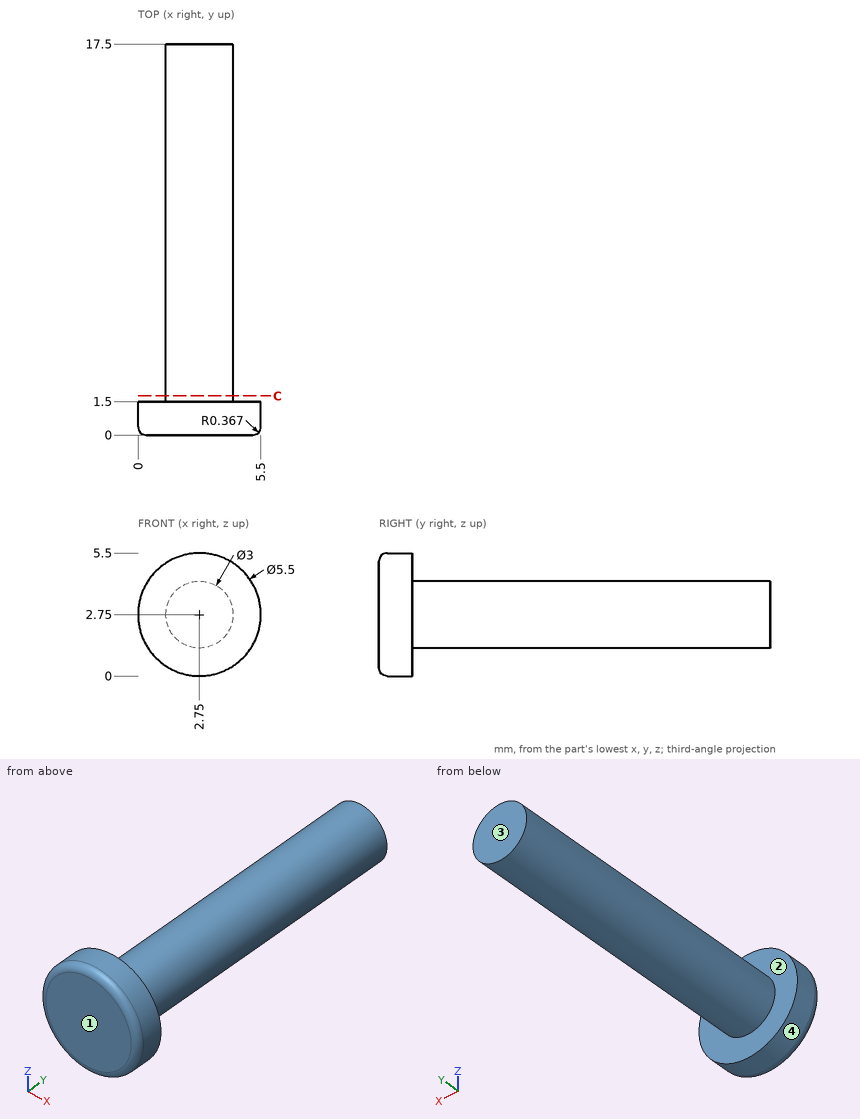
The figure shows three views and two pictorial views of one solid part (mm, origin at its lowest corner). Answer the questions. A direction names the side the tool comes from. Round coordinates to 2 decimals unless told otherwise and drop trailing zeros. Order: outer loops, then holes, each group sorted by start corner. A loop starts at its lowest first (then second) coordinate and runs counter-clockwise, first axis right, second up. Notation, with made-up numbers: M -1.75,58 L 19.25,58 A9 cw 19.25,74 Z; hole C 1,67 d11. An arc over 180 degrees is marked long. Answer in a Markdown table with one row per item. Add a question column.
1) Flat-ended cylindrical pins translate along their axes: pin 1 Ø3 at (y, z) = (2.5, 1) entering from +X; pin 2 Ø1 at (x, y) = (1.5, 11) entering from +Z. Find the tip coordinate at first contact, or state that the pin passes through.
2) The part is cut by section C-C on y = 1.75. Determine the outline of the cut face in (x, z).
3) Which of the six approach directions +Z, -Z, +X, -X, +Y, -Y give full straight-line access (tool end or side, diameter ignored) to the marked faces 1 and 2?
4) Determine the mould class of the marked faces 3 and 4 for opening direction Z: pulls with the +Z half, pulls with the -Z half, needs draft (parallel to the pull), parting line crosses it, or undercut.
5) Consider line 1 along Y through (x, z) = (1.5, 1.55); line 2 along Z through (x, y) = (2.6, 1.25); line 3 along Z through (x, y) = (2.75, 10). Determine where each line is inside the solid, lowest interval first. Write a range as from..to.
Findings below:
| question | item | result |
|---|---|---|
| 1 | pin 1 | stops at x = 5.43 |
| 1 | pin 2 | stops at z = 4.05 |
| 2 | outline | C 2.75,2.75 d3 |
| 3 | face 1 | +Z, -Z, +X, -X, -Y |
| 3 | face 2 | +Y |
| 4 | face 3 | needs draft |
| 4 | face 4 | parting line crosses it |
| 5 | line 1 | y = 0..1.5 |
| 5 | line 2 | z = 0..5.5 |
| 5 | line 3 | z = 1.25..4.25 |
